For this review, take the finished solid that the model builds, in its own axes (mm). A direction names the side the tool comes from. Round coordinates to 2 decimals unless told otherwise and drop trailing zeros. Loops run counter-clockwise (first coordinate to the right, second up) from the corner with the lowest first, then second, coordinate; pieces in that order, holes last.
1) Mouldability with a two-part tool opening along Z and no side actions: class faces 1 (the cylindrical face through (28, 14.1, 13)), 2 (the flat face through (-28, 13.7, 34)), 3 (the flat face through (-28, -17, 36)) as pulls with the +Z half, pulls with the -Z half, needs draft (parallel to the pull), parting line crosses it, or undercut.
2) Insertion check: pin 1 (1.8 mm diameter, centred on x = 28, y = 2, fed in from +Z); pin 2 (12 mm diameter, centred on x = -21, z = 32, fed in from +Y); pin 3 (8 mm diameter, centred on x = -11, y = -5, fed in from +Z); pin 4 (12 mm diameter, centred on x = 11.5, z = 14.5, fed in from +Y). Each pin has a flat end and moves straight along its axis. Give the tip position at first contact, or say it passes through.
3) Take a section at D-D (z = 8.5). State the section outline as (x, y) points.
4) Wall thickness on L1, parallel to X at y = 15, z = 12; L2, parallel to Z at x = 26.5, y = 2.5; L3, parallel to Y at x = 26, z = 34: over which ranges is each line inside the solid? List them lowest first.
5) Take a section at A-A (z = 33.5). State the section outline as (x, y) points.
6) Tool access review of faces 4 (the flat face through (-31, 0, 22)), 5 (the flat face through (28, -13.7, 34)), 6 (the cylindrical face through (28, -14.1, 19)): name each direction out of +Z, -Z, +X, -X, +Y, -Y from which nothing blocks a thin tool from reaching the whole face with its end or side.
7) Take a section at B-B (y = -7.5). State the section outline as (x, z) points, then the cut area to 3 significant figures.
Autodesk Inventor part; units mm, degrees
ref_plane "YZ Plane" through (0, 0, 0) normal (1, 0, 0) x (0, 1, 0)
ref_plane "XZ Plane" through (0, 0, 0) normal (0, 1, 0) x (-1, 0, 0)
ref_plane "XY Plane" through (0, 0, 0) normal (0, 0, 1) x (1, 0, 0)
sketch "スケッチ1" plane through (0, 0, 0) normal (0, 0, 1) x (1, 0, 0)
  line L0 (-31, 20) -> (31, 20)
  line L1 (31, 20) -> (31, -20)
  line L2 (31, -20) -> (-31, -20)
  line L3 (-31, -20) -> (-31, 20)
  line L4 (-31, 20) -> (31, -20) construction
  line L5 (31, 20) -> (-31, -20) construction
  point P0 (0, 0)
  dimension "d0" = 62
  dimension "d1" = 40
extrude "押し出し1" add sketch "スケッチ1" along normal blind 6
sketch "スケッチ2" plane through (0, 0, 6) normal (0, 0, 1) x (1, 0, 0)
  line L0 (31, 20) -> (-31, 20)
  line L1 (-31, -20) -> (31, -20)
  line L2 (-31, 20) -> (-25, 20)
  line L3 (-25, 20) -> (-25, -20)
  line L4 (-25, -20) -> (-31, -20)
  line L5 (-31, -20) -> (-31, 20)
  line L6 (31, -20) -> (31, 20)
  line L7 (31, 20) -> (25, 20)
  line L8 (25, 20) -> (25, -20)
  line L9 (25, -20) -> (31, -20)
  line L10 (31, -20) -> (31, 20)
  point P0 (0, 0)
  dimension "d4" = 6
  dimension "d5" = 6
extrude "押し出し2" add sketch "スケッチ2" along normal blind 30 contours L6 L1 L8 L0 | L3 L1 L5 L0
sketch "スケッチ3" plane through (31, -20, 0) normal (1, 0, 0) x (0, 0, -1)
  line L0 (-6, 0) -> (-36, 0)
  line L1 (-18.303, 0) -> (-8.303, 0)
  line L2 (0, 0) -> (0, 40)
  line L3 (-36, 0) -> (-36, 40)
  line L4 (-36, 0) -> (-17.2102, 0)
  line L5 (0, 0) -> (-16, 0)
  line L6 (-16, 0) -> (-16, 20)
  line L7 (-16, 20) -> (0, 20)
  line L8 (0, 20) -> (0, 0)
  line L9 (-20.25, 35.337) -> (-11.75, 35.337)
  line L10 (-11.75, 35.337) -> (-11.75, 4.663)
  line L11 (-11.75, 4.663) -> (-20.25, 4.663)
  line L12 (-20.25, 4.663) -> (-20.25, 35.337)
  line L13 (-20.25, 35.337) -> (-11.75, 4.663) construction
  line L14 (-11.75, 35.337) -> (-20.25, 4.663) construction
  line L15 (-40, 6.3) -> (-32, 6.3)
  line L16 (-32, 6.3) -> (-32, 33.7)
  line L17 (-32, 33.7) -> (-40, 33.7)
  line L18 (-40, 33.7) -> (-40, 6.3)
  line L19 (-40, 6.3) -> (-32, 33.7) construction
  line L20 (-32, 6.3) -> (-40, 33.7) construction
  point P0 (0, 20)
  point P1 (-36, 20)
  point P2 (-36, 33.7)
  point P3 (-36, 6.3)
  dimension "d9" = 36
  dimension "d10" = 40
  dimension "d11" = 20
  dimension "d12" = 16
  dimension "d13" = 8.5
  dimension "d17" = 8
  dimension "d18" = 27.4
extrude "押し出し3" cut sketch "スケッチ3" against normal blind 100 contours L3 L17 L16 L15 | L11 L12 L9 L10 L7 L6 | L6 L7 L10 L11
fillet "フィレット1" radius 4.25 8 edges at (28, 15.337, 11.75) (28, 15.337, 20.25) (28, -15.337, 11.75) (28, -15.337, 20.25) (-28, 15.337, 11.75) (-28, 15.337, 20.25) (-28, -15.337, 11.75) (-28, -15.337, 20.25)
equation "\"d5\" = d4"
equation "\"d11\" = 0.5 * d10"
properties part number "main"
Response:
1. face 1: undercut
1. face 2: needs draft
1. face 3: pulls with the +Z half
2. pin 1: stops at z = 32
2. pin 2: stops at y = 20
2. pin 3: stops at z = 6
2. pin 4: passes through
3. outline: (-31, -20) - (-25, -20) - (-25, 20) - (-31, 20) - close; (25, -20) - (31, -20) - (31, 20) - (25, 20) - close
4. L1: x = -31 to -25, 25 to 31
4. L2: z = 0 to 11.75, 20.25 to 32
4. L3: y = -20 to -13.7, 13.7 to 20
5. outline: (-31, -20) - (-25, -20) - (-25, -13.7) - (-31, -13.7) - close; (-31, 13.7) - (-25, 13.7) - (-25, 20) - (-31, 20) - close; (25, -20) - (31, -20) - (31, -13.7) - (25, -13.7) - close; (25, 13.7) - (31, 13.7) - (31, 20) - (25, 20) - close
6. face 4: +Z, -Z, -X, +Y, -Y
6. face 5: +Z, +X, -X
6. face 6: +X, -X
7. outline: (-31, 0) - (31, 0) - (31, 11.75) - (25, 11.75) - (25, 6) - (-25, 6) - (-25, 11.75) - (-31, 11.75) - close; (-31, 20.25) - (-25, 20.25) - (-25, 32) - (-31, 32) - close; (25, 20.25) - (31, 20.25) - (31, 32) - (25, 32) - close
7. area: 582 mm2
